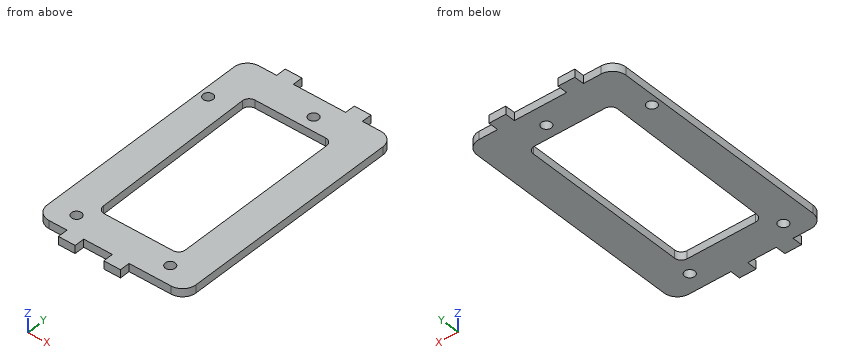
```python
from build123d import *

# Parameters (mm, degrees)
CROQUIS1_R              = 1.5
SALIENTE_EXTRUIR1_DEPTH = 2.4
CORTAR_EXTRUIR1_REACH   = 82.193
CROQUIS2_R              = 1.5


with BuildPart() as part:
    # Croquis1 → Saliente-Extruir1 (new body)
    with BuildSketch(Plane.XY):
        with BuildLine():
            Line((-27.735211809, 52.645866632), (-43.365211809, 52.645866632))
            Line((-43.365211809, 52.645866632), (-43.365211809, 55.645866632))
            Line((-43.365211809, 55.645866632), (-48.365211809, 55.645866632))
            Line((-48.365211809, 55.645866632), (-48.365211809, 52.645866632))
            Line((-48.365211809, 52.645866632), (-53.695211809, 52.645866632))
            ThreePointArc((-53.695211809, 52.645866632), (-56.523638933, 51.474293757), (-57.695211809, 48.645866632))
            Line((-57.695211809, 48.645866632), (-57.695211809, -16.854133368))
            ThreePointArc((-57.695211809, -16.854133368), (-56.523638933, -19.682560493), (-53.695211809, -20.854133368))
            Line((-53.695211809, -20.854133368), (-48.365211809, -20.854133368))
            Line((-48.365211809, -20.854133368), (-48.365211809, -23.854133368))
            Line((-48.365211809, -23.854133368), (-43.365211809, -23.854133368))
            Line((-43.365211809, -23.854133368), (-43.365211809, -20.854133368))
            Line((-43.365211809, -20.854133368), (-34.815211809, -20.854133368))
            Line((-34.815211809, -20.854133368), (-34.815211809, -23.854133368))
            Line((-34.815211809, -23.854133368), (-29.815211809, -23.854133368))
            Line((-29.815211809, -23.854133368), (-29.815211809, -20.854133368))
            Line((-29.815211809, -20.854133368), (-17.225211809, -20.854133368))
            ThreePointArc((-17.225211809, -20.854133368), (-14.396784684, -19.682560493), (-13.225211809, -16.854133368))
            Line((-13.225211809, -16.854133368), (-13.225211809, 48.645866632))
            ThreePointArc((-13.225211809, 48.645866632), (-14.396784684, 51.474293757), (-17.225211809, 52.645866632))
            Line((-17.225211809, 52.645866632), (-22.735211809, 52.645866632))
            Line((-22.735211809, 52.645866632), (-22.735211809, 55.645866632))
            Line((-22.735211809, 55.645866632), (-27.735211809, 55.645866632))
            Line((-27.735211809, 55.645866632), (-27.735211809, 52.645866632))
        make_face()
        with Locations((-55.195211809, 36.645866632)):
            Circle(CROQUIS1_R, mode=Mode.SUBTRACT)
        with Locations((-50.195211809, -15.354133368)):
            Circle(CROQUIS1_R, mode=Mode.SUBTRACT)
        with Locations((-22.195211809, -15.354133368)):
            Circle(CROQUIS1_R, mode=Mode.SUBTRACT)
        with BuildLine():
            Line((-35.550211809, 42.645866632), (-25.225211809, 42.645866632))
            ThreePointArc((-25.225211809, 42.645866632), (-23.810998246, 42.060080194), (-23.225211809, 40.645866632))
            Line((-23.225211809, 40.645866632), (-23.225211809, -8.854133368))
            ThreePointArc((-23.225211809, -8.854133368), (-23.810998246, -10.26834693), (-25.225211809, -10.854133368))
            Line((-25.225211809, -10.854133368), (-45.720101709, -10.854133368))
            ThreePointArc((-45.720101709, -10.854133368), (-47.125432715, -10.277174044), (-47.719944893, -8.879178133))
            Line((-47.719944893, -8.879178133), (-48.339851435, 40.620821867))
            ThreePointArc((-48.339851435, 40.620821867), (-47.763048927, 42.051197638), (-46.340008251, 42.645866632))
            Line((-46.340008251, 42.645866632), (-35.550211809, 42.645866632))
        make_face(mode=Mode.SUBTRACT)
    extrude(amount=SALIENTE_EXTRUIR1_DEPTH)

    # Croquis2 → Cortar-Extruir1 (cut, up to next)
    with BuildSketch(Plane.XY.offset(2.4), mode=Mode.PRIVATE) as cortar_extruir1_sk1:
        with Locations((-32.195211809, 46.645866632)):
            Circle(CROQUIS2_R)
    cortar_extruir1_tool1 = extrude(cortar_extruir1_sk1.sketch, amount=-CORTAR_EXTRUIR1_REACH, mode=Mode.PRIVATE) & part.part
    add(cortar_extruir1_tool1.solids().sort_by_distance((-32.195212, 46.645867, 2.4))[0], mode=Mode.SUBTRACT)


solid = part.part
```
Work out the finished part from the listing and answer in its coordinate system (mm). Coordinates: 2 decimals unless noted, no trailing zeros. Write each loop counter-clockwise with the first axis right and the second up, starting at its lowest first coordinate (ties: lowest second). Pieces come first, ordered by that corner, then holes.
Q1. A cutting plane is placed at D-D, the plane z = 0.65. State how many separate pieces and enclosed holes the cut face has, then the cut area to 3 significant figures.
Q2. A cutting plane is placed at C-C, the plane x = -18.5. Give the vertices of the cut face in (y, z).
Q3. A cutting plane is placed at A-A, the plane x = -40. Give the vertices of the cut face in (y, z).
Q4. Each of these flat-tipped pins is pushed along its axis until it touches: pin 1 Ø1.2 at (x, z) = (-35.5, 0.5) entering from +Y; pin 2 Ø0.7 at (y, z) = (54.5, 0.5) entering from -X; pin 3 Ø2.5 at (x, y) = (-22.2, -15.35) entering from -Z; pin 4 Ø1.2 at (x, z) = (-40, 1.5) entering from -Y. Where does it stop, or does it pass through?
Q5. A cutting plane is placed at B-B, the plane y = -2.5. Give the vertices of the cut face in (x, z).
Q6. Find the intervals of material crossed by line 1 (Y direction, x = -27.5, z = 1.15); line 2 (Y direction, x = -32.5, z = 0.5); line 3 (X direction, y = -14.5, z = 2.15), in increasing order.
Findings below:
1. separate pieces: 1
1. enclosed holes: 5
1. area: 1,960 mm2
2. outline: (-20.85, 0) - (52.65, 0) - (52.65, 2.4) - (-20.85, 2.4) - close
3. outline: (-20.85, 0) - (-10.85, 0) - (-10.85, 2.4) - (-20.85, 2.4) - close; (42.65, 0) - (52.65, 0) - (52.65, 2.4) - (42.65, 2.4) - close
4. pin 1: stops at y = 52.65
4. pin 2: stops at x = -48.37
4. pin 3: passes through
4. pin 4: stops at y = -20.85
5. outline: (-57.7, 0) - (-47.8, 0) - (-47.8, 2.4) - (-57.7, 2.4) - close; (-23.23, 0) - (-13.23, 0) - (-13.23, 2.4) - (-23.23, 2.4) - close
6. line 1: y = -20.85 to -10.85, 42.65 to 55.65
6. line 2: y = -23.85 to -10.85, 42.65 to 45.18, 48.11 to 52.65
6. line 3: x = -57.7 to -51.43, -48.96 to -23.43, -20.96 to -13.23
